Autodesk Fusion 360 part; units mm, degrees
sketch "Sketch1" plane through (0, 0, 0) normal (0, 1, 0) x (1, 0, 0)
  line L0 (140, -17.5) -> (-140, -17.5)
  line L1 (-140, -17.5) -> (-140, 17.5)
  line L2 (-140, 17.5) -> (140, 17.5)
  line L3 (140, 17.5) -> (140, -17.5)
  line L4 (140, -17.5) -> (-140, 17.5) construction
  line L5 (-140, -17.5) -> (140, 17.5) construction
  line L6 (150, -27.5) -> (-150, -27.5)
  line L7 (-150, -27.5) -> (-150, 27.5)
  line L8 (-150, 27.5) -> (150, 27.5)
  line L9 (150, 27.5) -> (150, -27.5)
  line L10 (150, -27.5) -> (-150, 27.5) construction
  line L11 (-150, -27.5) -> (150, 27.5) construction
  dimension "d1" = 280
  dimension "d2" = 35
  dimension "d3" = 300
  dimension "d4" = 55
extrude "Extrude1" add sketch "Sketch1" along normal blind 2
sketch "Sketch2" plane through (0, 0, 27.5) normal (0, 0, 1) x (1, 0, 0)
  line L0 (-150, 0) -> (150, 0)
  line L1 (150, 0) -> (150, 2)
  line L2 (150, 2) -> (-150, 2)
  line L3 (-150, 2) -> (-150, 0)
extrude "Extrude2" add sketch "Sketch2" along normal blind 20
move_face "OffsetFaces1" offset 25 1 faces at (-150, 0.6667, 22.5)
sketch "Sketch3" plane through (0, 0, 0) normal (0, 1, 0) x (1, 0, 0)
  line L0 (155, -50) -> (0, -50)
  line L1 (0, -50) -> (0, 50)
  line L2 (0, 50) -> (155, 50)
  line L3 (155, 50) -> (155, -50)
extrude "Extrude3" cut sketch "Sketch3" along normal blind 60
fillet "Fillet1" radius 10 1 edges at (-175, 1, 47.5)
fillet "Fillet2" radius 10 1 edges at (-175, 1, -27.5)
move_face "OffsetFaces2" offset -10 1 faces at (-46.6667, 0.6667, 17.5)
move_face "OffsetFaces3" offset 10 1 faces at (-93.3333, 0.6667, -17.5)
hole "Hole1" at (-164.3594, 2, 10.5834) direction (0, -1, 0) diameter 3 depth 5 tip angle 118
hole "Hole2" at (-24.6611, 2, 36.9776) direction (0, -1, 0) diameter 3 depth 5 tip angle 118
hole "Hole3" at (-24.9224, 2, -18.284) direction (0, -1, 0) diameter 3 depth 5 tip angle 118
Part model, mm, in its own coordinate system. Coordinates: 2 decimals unless noted, no trailing zeros. Loops run counter-clockwise (first coordinate to the right, second up) from the corner with the lowest first, then second, coordinate; pieces in that order, holes last. Notation, with made-up numbers: M 5,42.5 L 38,42.5 A30 cw 38,66.5 Z; hole C -30,24.5 d1. An arc over 180 degrees is marked long. Use a Markdown table: item, result. Add a question column.
Q1. Mould opens along X. For faces 1 (the cylindrical face through (-172.15, 1.01, 44.49)), 2 (the flat face through (-108, 0, -16)), 3 (the cylindrical face through (-25.11, 0.99, 38.41)) say: +X half, -X half, draft (parallel to the pull), parting line (faces both ways), or undercut.
Q2. Cut at A-A (x = -119.5). Write the cut outline in (y, z).
Q3. Cut at B-B (y = 0.9). Write the cut outline in (x, z).
Q4. Pin check, flat tips, straight feed: P1, Ø10, axis at x = -110, z = 19.5, coming from the -Y side; P2, Ø0.6, axis at y = 1, z = 13, coming from the +X side. Stop position of each tip, or through.
Q5. Probe L1, parallel to Z at x = -71.5, y = 1; L2, parallel to X at y = 0.3, z = 16.5; L3, parallel to X at y = 1.45, z = -18. List the from-to ranges inside material, lowest first.
Q6. Cut at C-C (z = 1.5). Write the cut outline in (x, y), and give its area (3 significant figures).
Worked out:
| question | item | result |
|---|---|---|
| 1 | face 1 | -X half |
| 1 | face 2 | draft |
| 1 | face 3 | undercut |
| 2 | outline | M 0,-27.5 L 2,-27.5 L 2,-7.5 L 0,-7.5 Z; M 0,27.5 L 2,27.5 L 2,47.5 L 0,47.5 Z |
| 3 | outline | M -175,-17.5 A10 ccw -165,-27.5 L 0,-27.5 L 0,-7.5 L -140,-7.5 L -140,27.5 L 0,27.5 L 0,47.5 L -165,47.5 A10 ccw -175,37.5 Z; hole C -164.36,10.58 d3; hole C -24.92,-18.28 d3; hole C -24.66,36.98 d3 |
| 4 | P1 | passes through |
| 4 | P2 | stops at x = -140 |
| 5 | L1 | z = -27.5 to -7.5, 27.5 to 47.5 |
| 5 | L2 | x = -175 to -140 |
| 5 | L3 | x = -174.99 to -26.4, -23.45 to 0 |
| 6 | outline | M -175,0 L -140,0 L -140,2 L -175,2 Z |
| 6 | area | 70.0 mm2 |
